from build123d import *

# Parameters (mm, degrees)
F0_W     = 5
F0_H     = 6
F1_DEPTH = 7.5
F2_R     = 1.5
F3_DEPTH = 4
F4_R     = 1.5
F5_DEPTH = 4


with BuildPart() as f1:
    # F0 (on Top) → F1 (new body)
    with BuildSketch(Plane.XY):
        with Locations((7.5, 16)):
            Rectangle(F0_W, F0_H)
        Polygon((2, 13), (0, 0), (15, 0), (13, 13), (10, 13), (5, 13), align=None)
    extrude(amount=F1_DEPTH)

    # F2 (on face) → F3 (cut)
    with BuildSketch(Plane(origin=(14.653179, 2.254335, 0), x_dir=(-0.152057, 0.988372, 0), z_dir=(0.988372, 0.152057, 0))):
        with Locations((9.319803, 4.095583)):
            Circle(F2_R)
    extrude(amount=-F3_DEPTH, mode=Mode.SUBTRACT)

    # F4 (on face) → F5 (cut)
    with BuildSketch(Plane(origin=(0, 0, 0), x_dir=(-0.152057, -0.988372, 0), z_dir=(-0.988372, 0.152057, 0))):
        with Locations((-11.632966, 3.637236)):
            Circle(F4_R)
    extrude(amount=-F5_DEPTH, mode=Mode.SUBTRACT)


solid = f1.part
Input: part model. Units: mm. Frame: model coordinates. A direction names the side the tool comes from. Give positions to 0.01 mm unless a question says otherwise; leave off trailing zeros. Loops run counter-clockwise (first coordinate to the right, second up) from the corner with the lowest first, then second, coordinate; pieces in that order, holes last. Notation, with made-up numbers: M 8,46.25 L 18,46.25 A23 ccw 18,78.25 Z; hole C -27.75,77.5 d6. An arc over 180 degrees is marked long. Use one line per item in the form item = value.
1. Section query A-A, the plane z = 0.5. Return the cut outline in (x, y).
Numbers:
outline = M 0,0 L 15,0 L 13,13 L 10,13 L 10,19 L 5,19 L 5,13 L 2,13 Z
2. Section query D-D, the plane z = 3.25. Return the cut outline in (x, y).
Numbers:
outline = M 0,0 L 15,0 L 13.42,10.24 L 9.47,9.63 L 9.09,12.08 L 13.05,12.69 L 13,13 L 10,13 L 10,19 L 5,19 L 5,13 L 2,13 L 1.99,12.93 L 5.94,12.32 L 5.5,9.46 L 1.55,10.07 Z
3. First-contact query: pin 1 (3 mm diameter, centred on y = 11.5, z = 3.5, fed in from -X); pin 2 (1.5 mm diameter, centred on x = 4, z = 4, fed in from +Y); pin 3 (1.8 mm diameter, centred on y = 16.5, z = 5.5, fed in from -X). Flat tips, straight axial feed; report the tip coordinate or a pass-through.
Numbers:
pin_1 = 1.54
pin_2 = 13
pin_3 = 5
4. Pull-direction query (X, two-part tool) for faces 5 (the face through (5.726, 10.91, 3.658)), 6 (the face through (10, 16, 4)), 7 (the face through (3.767, 11.519, 2.173)), 8 (the face through (5, 16, 4)); classes: released by +X, released by -X, zero draft, split by the parting line, or undercut.
Numbers:
face_5 = undercut
face_6 = released by +X
face_7 = undercut
face_8 = released by -X
5. Line query: L1, parallel to X at y = 13.25, z = 5.5; L2, parallel to Z at x = 5.25, y = 11.25; L3, parallel to Z at x = 4.5, y = 10.5. Output: solid intervals per line, ascending.
Numbers:
L1 = 5 to 10
L2 = 0 to 2.16, 5.11 to 7.5
L3 = 0 to 2.25, 5.02 to 7.5
6. Reachability of faces 1 (the face through (4, 13, 4)), 2 (the face through (12, 13, 4)), 3 (the face through (9.286, 10.837, 4.117)), 4 (the face through (7, 19, 4)) from +Z, -Z, +X, -X, +Y, -Y: full face, straight path, thin tool, end or side. Return the list, or none.
Numbers:
face_1 = +Z, -Z, -X, +Y
face_2 = +Z, -Z, +X, +Y
face_3 = none
face_4 = +Z, -Z, +X, -X, +Y
7. Section query C-C, the plane x = 14.25. Return the cut outline in (y, z) (3 decimals).
Numbers:
outline = M 0,0 L 4.875,0 L 4.875,7.5 L 0,7.5 Z
8. Section query B-B, the plane y = 15.5. Return the cut outline in (x, z).
Numbers:
outline = M 5,0 L 10,0 L 10,7.5 L 5,7.5 Z
